Geometry check sheet. Reference: the model listing, model coordinates, mm. A direction names the side the tool comes from. Round coordinates to 2 decimals unless told otherwise and drop trailing zeros. Write each loop counter-clockwise with the first axis right and the second up, starting at its lowest first coordinate (ties: lowest second). Pieces come first, ordered by that corner, then holes.
Item 1: Cross-section at A-A (y = 11). Enter the section's corners in (x, z) (3 decimals), then the cut area to 3 significant figures.
Item 2: Draft check along Z on faces 5 (the face through (-55.015, 26.479, -0.66)), 6 (the face through (-76, 28, 6)), 7 (the face through (1.08, 47.42, 4.88)). Enter one of: pulls with the +Z half, pulls with the -Z half, needs draft (parallel to the pull), parting line crosses it, or undercut.
Item 3: Access from +Z, -Z, +X, -X, +Y, -Y to the whole of each face (thin tool, end or side, straight path). Record for faces 1 (the face through (-9, 51, -12)), 2 (the face through (0, 42, 55)), 3 (the face through (5.2, 42, 0.1)), 4 (the face through (57, 5, 1)).
Item 4: Cross-section at C-C (y = 35). Enter the section's corners in (x, z), then the cut area to 3 significant figures.
Item 5: Cross-section at B-B (x = 0). Enter the section's corners in (y, z), then the cut area to 3 significant figures.
Item 6: Cross-section at D-D (z = 0). State how many separate pieces and enclosed holes the cut face has, then the cut area to 3 significant figures.
Item 7: Depth check by flat-ended pin: P1, Ø10, axis at y = 35, z = 25.5, coming from the -X side; P2, Ø6, axis at x = 70, y = 10, coming from the -Z side; P3, Ø16, axis at x = 57.5, y = 12, coming from the +Z side; P4, Ø9, axis at x = 0, z = 0, coming from the -Y side. Enter the tip coordinate at first touch or a pass-through.
Item 8: Scan lines: probe 1 along Z at (x, y) = (70, 21.5); probe 2 along X at (y, z) = (20, 1); probe 3 along Y at (x, z) = (-49, -9). Record each from-to range of solid material in increasing order.
from build123d import *

# Parameters (mm, degrees)
BOSS_EXTRUDE1_DEPTH      = 55
SKETCH4_W                = 180
SKETCH4_H                = 20
BOSS_EXTRUDE2_DEPTH      = 50
CUT_EXTRUDE1_REACH       = 152.665
SKETCH5_W                = 45
SKETCH5_H                = 5
CUT_EXTRUDE2_REACH       = 152.665
SKETCH7_R                = 15
BOSS_EXTRUDE3_DEPTH      = 3
HOLE1_D                  = 16
BOSS_EXTRUDE4_REACH      = 120.042
BOSS_EXTRUDE4_END_RADIUS = 50
SKETCH10_R               = 15
HOLE2_D                  = 10
SKETCH13_R               = 8
CUT_EXTRUDE3_DEPTH       = 42


with BuildPart() as part:
    # Sketch2 → Boss-Extrude1 (new, symmetric)
    with BuildSketch(Plane.XY):
        with BuildLine():
            Line((-50, 0), (50, 0))
            ThreePointArc((50, 0), (0, 50), (-50, 0))
        make_face()
    extrude(amount=BOSS_EXTRUDE1_DEPTH, both=True)

    # Sketch4 → Boss-Extrude2 (add, symmetric)
    with BuildSketch(Plane.XY):
        with Locations((0, 15)):
            Rectangle(SKETCH4_W, SKETCH4_H)
    extrude(amount=BOSS_EXTRUDE2_DEPTH, both=True)

    # Sketch5 → Cut-Extrude1 (cut, up to next)
    with BuildSketch(Plane.XY.offset(55), mode=Mode.PRIVATE) as cut_extrude1_sk1:
        with Locations((67.5, 2.5)):
            Rectangle(SKETCH5_W, SKETCH5_H)
    cut_extrude1_tool1 = extrude(cut_extrude1_sk1.sketch, amount=-CUT_EXTRUDE1_REACH, mode=Mode.PRIVATE) & part.part
    cut_extrude1 = cut_extrude1_tool1.solids().sort_by_distance((67.5, 2.5, 55))[0]
    add(cut_extrude1, mode=Mode.SUBTRACT)

    # Mirror1: Cut-Extrude1 across plane
    add(cut_extrude1.mirror(Plane(origin=(0, 0, 0), x_dir=(0, 0, 1), z_dir=(1, 0, 0))), mode=Mode.SUBTRACT)

    # Sketch6 → Cut-Extrude2 (cut, up to next)
    with BuildSketch(Plane.XY.offset(55), mode=Mode.PRIVATE) as cut_extrude2_sk1:
        with BuildLine():
            Line((-40, 0), (40, 0))
            ThreePointArc((40, 0), (0, 40), (-40, 0))
        make_face()
    cut_extrude2_tool1 = extrude(cut_extrude2_sk1.sketch, amount=-CUT_EXTRUDE2_REACH, mode=Mode.PRIVATE) & part.part
    add(cut_extrude2_tool1.solids().sort_by_distance((0, 16.976527, 55))[0], mode=Mode.SUBTRACT)

    # Sketch7 → Boss-Extrude3 (add)
    with BuildSketch(Plane(origin=(0, 25, 0), x_dir=(1, 0, 0), z_dir=(0, 1, 0))):
        with Locations((70, 0)):
            Circle(SKETCH7_R)
    boss_extrude3 = extrude(amount=BOSS_EXTRUDE3_DEPTH)

    # Mirror2: Boss-Extrude3 across plane
    add(boss_extrude3.mirror(Plane(origin=(0, 0, 0), x_dir=(0, 0, 1), z_dir=(1, 0, 0))))

    # Hole1 (through all)
    with Locations(Plane(origin=(0, 28, 0), x_dir=(1, 0, 0), z_dir=(0, 1, 0))):
        with Locations((70, 0), (-70, 0)):
            Hole(HOLE1_D / 2)

    # Boss-Extrude4: up to this cylinder (the profile starts outside it)
    boss_extrude4_end = Plane(origin=(0, 0, 0), z_dir=(0, 0, -1)) * Cylinder(BOSS_EXTRUDE4_END_RADIUS, 341.084, mode=Mode.PRIVATE)
    # Sketch10 → Boss-Extrude4 (add, up to the surface)
    with BuildSketch(Plane(origin=(0, 53, 0), x_dir=(1, 0, 0), z_dir=(0, 1, 0)), mode=Mode.PRIVATE) as boss_extrude4_sk1:
        with Locations(Location((0, 0, 0), (0, 0, 270))):
            Circle(SKETCH10_R)
    boss_extrude4_tool1 = extrude(boss_extrude4_sk1.sketch, amount=-BOSS_EXTRUDE4_REACH, mode=Mode.PRIVATE) - boss_extrude4_end
    add(boss_extrude4_tool1.solids().sort_by_distance((0, 53, 0))[0])

    # Hole2 (through all)
    with Locations(Plane(origin=(0, 53, 0), x_dir=(1, 0, 0), z_dir=(0, 1, 0))):
        with Locations((0, 0)):
            Hole(HOLE2_D / 2)

    # Sketch13 → Cut-Extrude3 (cut)
    with BuildSketch(Plane(origin=(0, 0, 0), x_dir=(1, 0, 0), z_dir=(0, 1, 0))):
        with Locations(Location((0, 0, 0), (0, 0, 90))):
            Circle(SKETCH13_R)
    extrude(amount=CUT_EXTRUDE3_DEPTH, mode=Mode.SUBTRACT)


solid = part.part
Resolved:
1. outline: (-90, -50) - (-48.775, -50) - (-48.775, -55) - (-38.458, -55) - (-38.458, 55) - (-48.775, 55) - (-48.775, 50) - (-90, 50) - close; (38.458, -55) - (48.775, -55) - (48.775, -50) - (90, -50) - (90, 50) - (48.775, 50) - (48.775, 55) - (38.458, 55) - close; hole circle Ø16 at (-70, 0); hole circle Ø16 at (70, 0)
1. area: 10,100 mm2
2. face 5: parting line crosses it
2. face 6: needs draft
2. face 7: undercut
3. face 1: +Y
3. face 2: +Z, +X, -X, +Y, -Y
3. face 3: -Y
3. face 4: +Z, -Z, +X, -Y
4. outline: (-35.71, -55) - (-19.36, -55) - (-19.36, 55) - (-35.71, 55) - close; (19.36, -55) - (35.71, -55) - (35.71, 55) - (19.36, 55) - close
4. area: 3,600 mm2
5. outline: (40, -55) - (50, -55) - (50, -15) - (53, -15) - (53, -5) - (42, -5) - (42, -8) - (40, -8) - close; (40, 8) - (42, 8) - (42, 5) - (53, 5) - (53, 15) - (50, 15) - (50, 55) - (40, 55) - close
5. area: 1,050 mm2
6. separate pieces: 4
6. enclosed holes: 0
6. area: 2,480 mm2
7. P1: stops at x = -40
7. P2: stops at z = -50
7. P3: stops at z = 50
7. P4: passes through
8. probe 1: z = -50 to -8, 8 to 50
8. probe 2: x = -90 to -77.94, -62.06 to -34.64, 34.64 to 62.06, 77.94 to 90
8. probe 3: y = 5 to 25
